from build123d import *

# Parameters (mm, degrees)
F0_R     = 58.9929104122
F4_DEPTH = 82.4266280979
F4_TAPER = -5
F1_R     = 12.7
F2_T     = -5.08


with BuildPart() as f4:
    # F0 (on Front) → F4 (new body)
    with BuildSketch(Plane.XZ):
        with Locations((0, 46.2810769677)):
            Circle(F0_R)
    extrude(amount=F4_DEPTH, taper=F4_TAPER)

    # F1
    f1_edges = [f4.edges().sort_by_distance(p)[0] for p in [
        (-58.99291, 0, 46.281077),
    ]]
    fillet(f1_edges, radius=F1_R)

    # F2
    f2_openings = [f4.faces().sort_by_distance(p)[0] for p in [
        (0, -82.426628, 46.281077),
    ]]
    offset(amount=F2_T, openings=f2_openings, kind=Kind.INTERSECTION)


solid = f4.part
For this review, take the finished solid that the model builds, in its own axes (mm). Round coordinates to 2 decimals unless told otherwise and drop trailing zeros. Order: outer loops, then holes, each group sorted by start corner. A loop starts at its lowest first (then second) coordinate and runs counter-clockwise, first axis right, second up. Notation, with made-up numbers: M 20,38 L 70,38 A18 cw 70,45 Z; hole C 6,48 d1. An arc over 180 degrees is marked long. Use a Markdown table: item, result. Add a question column.
Item 1: Mouldability with a two-part tool opening along X and no side actions: class faces 1 (the flat face through (-1, -5.08, 47)), 2 (the conical face through (-8.13, -39.64, 108.21)), 3 (the flat face through (-1, 0, 47)) as released by +X, released by -X, zero draft, split by the parting line, or undercut.
Item 2: Add section C-C, the plane y = -64.5. Give the boundary of the cut face in (x, z).
Item 3: Add section A-A, the plane x = 0. Give the boundary of the cut face in (y, z), then the cut area to 3 significant figures.
Item 4: To check wall thickness, follow line 1 along Y through (x, z) = (-5, 46); line 2 along Z through (x, y) = (27, -53.5); line 3 along X through (y, z) = (-24, 34.5). State the ranges of each line that lie inside material, in increasing order.
Item 5: Insertion check: pin 1 (10 mm diameter, centred on y = -22.5, z = 10, fed in from +X); pin 2 (4 mm diameter, centred on x = -13.5, z = 96, fed in from +Y); pin 3 (8 mm diameter, centred on x = -3.5, y = -68.5, fed in from +Z). Each pin has a flat end and moves straight along its axis. Give the tip position at first contact, or say it passes through.
Item 6: Add section B-B, the plane y = -73. Give the boundary of the cut face in (x, z).
Geometry results:
| question | item | result |
|---|---|---|
| 1 | face 1 | undercut |
| 1 | face 2 | split by the parting line |
| 1 | face 3 | zero draft |
| 2 | outline | C 0,46.28 d129.27; hole C 0,46.28 d119.07 |
| 3 | outline | M -82.43,-19.92 L -11.59,-13.73 A12.7 ccw 0,-1.07 L 0,93.64 A12.7 ccw -11.59,106.29 L -82.43,112.49 L -82.43,107.39 L -12.04,101.23 A7.62 cw -5.08,93.64 L -5.08,-1.07 A7.62 cw -12.04,-8.67 L -82.43,-14.82 Z |
| 3 | area | 1,350 mm² |
| 4 | line 1 | y = -5.08 to 0 |
| 4 | line 2 | z = -11.38 to -5.7, 98.26 to 103.95 |
| 4 | line 3 | x = -59.95 to -54.74, 54.74 to 59.95 |
| 5 | pin 1 | stops at x = 52.37 |
| 5 | pin 2 | stops at y = -0.19 |
| 5 | pin 3 | stops at z = 111.56 |
| 6 | outline | C 0,46.28 d130.76; hole C 0,46.28 d120.56 |
